```python
from build123d import *

# Parameters (mm, degrees)
F0_W     = 72
F0_H     = 20
F1_DEPTH = 5
F2_W     = 14
F2_H     = 20
F3_DEPTH = 3.5
F4_R     = 3
F5_DEPTH = 3.5


with BuildPart() as f1:
    # F0 (on Top) → F1 (new body)
    with BuildSketch(Plane.XY):
        Rectangle(F0_W, F0_H)
    extrude(amount=F1_DEPTH)

    # F2 (on face) → F3 (cut)
    with BuildSketch(Plane.XY.offset(5)):
        with Locations((27, 0)):
            Rectangle(F2_W, F2_H)
        with Locations((-27, 0)):
            Rectangle(F2_W, F2_H)
    extrude(amount=-F3_DEPTH, mode=Mode.SUBTRACT)

    # F4 (on face) → F5 (join)
    with BuildSketch(Plane.XY.offset(1.5)):
        with Locations((-27, 0)):
            Circle(F4_R)
        with Locations((27, 0)):
            Circle(F4_R)
    extrude(amount=F5_DEPTH)


solid = f1.part
```
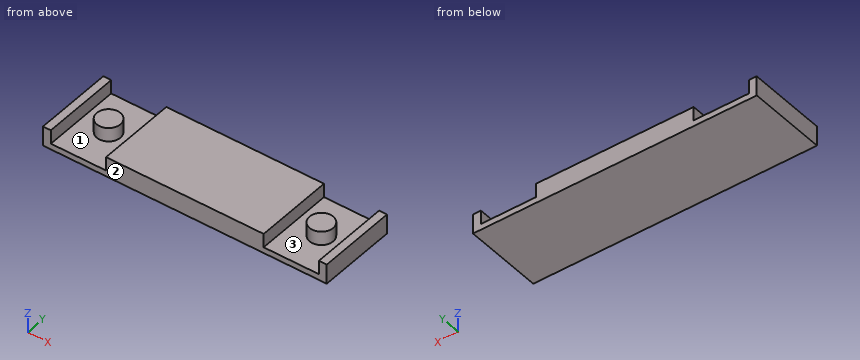
Check sheet for the modelled part. Datum: model origin and axes. Units: mm. Face numbers are marked on the shaded views. Round coordinates to 2 decimals unless told otherwise and drop trailing zeros. Write each loop counter-clockwise with the first axis right and the second up, starting at its lowest first coordinate (ties: lowest second). Pieces come first, ordered by that corner, then holes. Notation, with made-up numbers: (39, 38) -> (85, 38) arc R21 ccw to (85, 55) -> close; hole circle Ø10 at (85.5, 64). An arc over 180 degrees is marked (long way). One line per question, with ' | ' between items. Start each with the question number.
1. Sectioned sample at B-B, the plane x = -27. Record the cut outline in (y, z).
2. Release check for a two-part mould opening along X. For the marked faces 1, 2 and 3 record: +X half, -X half, draft (parallel to the pull), parting line (faces both ways), or undercut.
3. Sectioned sample at A-A, the plane z = 2.3. Record the cut outline in (x, y).
4. Sectioned sample at C-C, the plane y = 5.75. Record the cut outline in (x, z), then the cut area to 3 significant figures.
5. Sectioned sample at D-D, the plane y = 0. Record the cut outline in (x, z), then the cut area to 3 significant figures.
6. Scan lines: line 1 along X through (y, z) = (-9, 3.05); line 2 along Y through (x, z) = (-27, 3.15); line 3 along Z through (x, y) = (28, 8.5). Record each from-to range of solid material in increasing order. Write a range as from..to.
Taken from the geometry:
1) outline: (-10, 0) -> (10, 0) -> (10, 1.5) -> (3, 1.5) -> (3, 5) -> (-3, 5) -> (-3, 1.5) -> (-10, 1.5) -> close
2) face 1: undercut | face 2: draft | face 3: undercut
3) outline: (-36, -10) -> (-34, -10) -> (-34, 10) -> (-36, 10) -> close; circle Ø6 at (-27, 0); (-20, -10) -> (20, -10) -> (20, 10) -> (-20, 10) -> close; circle Ø6 at (27, 0); (34, -10) -> (36, -10) -> (36, 10) -> (34, 10) -> close
4) outline: (-36, 0) -> (36, 0) -> (36, 5) -> (34, 5) -> (34, 1.5) -> (20, 1.5) -> (20, 5) -> (-20, 5) -> (-20, 1.5) -> (-34, 1.5) -> (-34, 5) -> (-36, 5) -> close | area: 262 mm^2
5) outline: (-36, 0) -> (36, 0) -> (36, 5) -> (34, 5) -> (34, 1.5) -> (30, 1.5) -> (30, 5) -> (24, 5) -> (24, 1.5) -> (20, 1.5) -> (20, 5) -> (-20, 5) -> (-20, 1.5) -> (-24, 1.5) -> (-24, 5) -> (-30, 5) -> (-30, 1.5) -> (-34, 1.5) -> (-34, 5) -> (-36, 5) -> close | area: 304 mm^2
6) line 1: x = -36..-34, -20..20, 34..36 | line 2: y = -3..3 | line 3: z = 0..1.5
